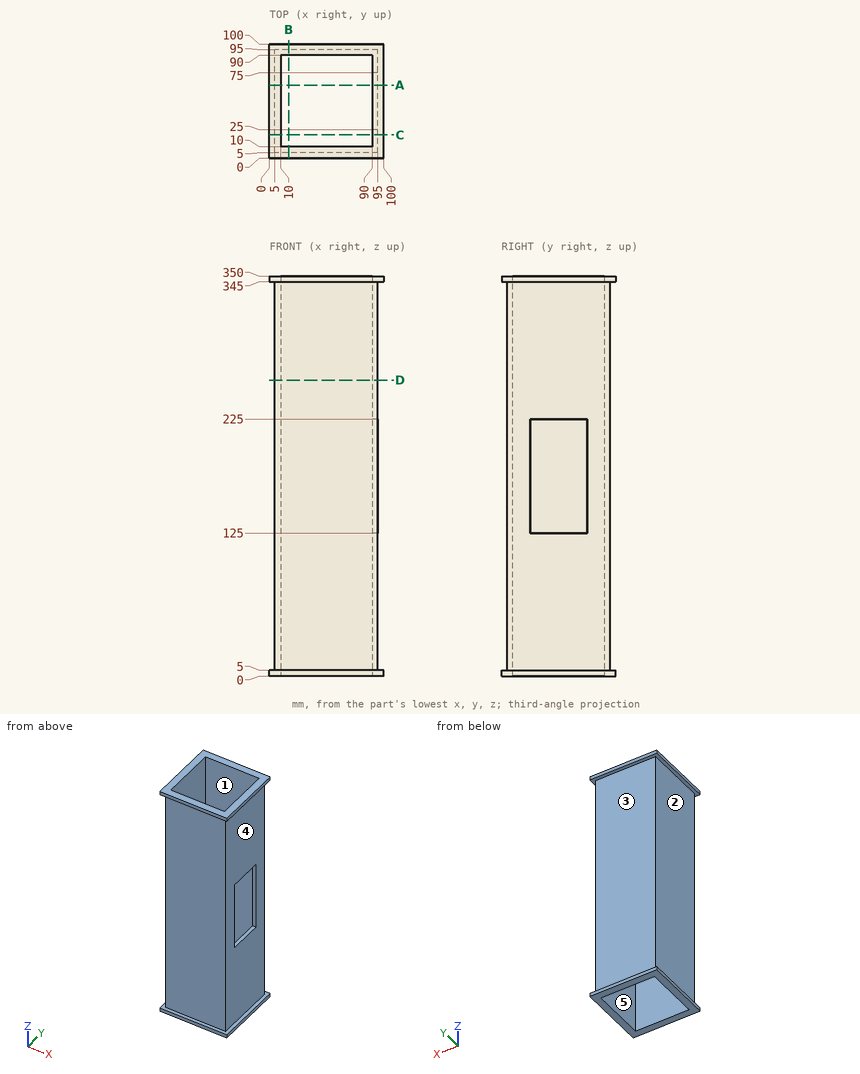
Job drawing, mm, ordinate dimensions from the low corner. One solid piece. A direction names the side the tool comes from. Give positions to 0.01 mm unless a question says otherwise; leave off trailing zeros. Loops run counter-clockwise (first coordinate to the right, second up) from the corner with the lowest first, then second, coordinate; pieces in that order, holes last. Notation, with made-up numbers: M 46,-31.75 L 69,-31.75 A13 ccw 69,-26.75 Z; hole C -5,67.25 d10. An arc over 180 degrees is marked long. Put each result on its own line as item: value. Start each with the question number.
1) Saw through at A-A (y = 64). List the corners of the cut face in (x, z), then the cut area to 3 significant figures.
2) Probe probe 1 along Z at (x, y) = (92, 42.5); probe 2 along Y at (x, z) = (37, 218.5). List the from-to ranges inside material, lowest first.
3) Pull direction Z, two halves, no side cores. Call the marked faces 4 and 5: +Z half, -Z half, draft (parallel to the pull), parting line (faces both ways), or undercut.
4) Saw through at B-B (x = 17). List the corners of the cut face in (y, z).
5) 3-axis set-ups, long thin cutter, end or side, ignore diameter. For the marked faces 1, 2 and 3: which of +Z, -Z, +X, -X, +Y, -Y reach the whole face in a straight line?
6) Flat gauge pins, fed straight in: pin 1 (2 mm diameter, centred on x = 35, z = 114, fed in from +Y); pin 2 (10 mm diameter, centred on y = 51.5, z = 245.5, fed in from -X); pin 3 (1.5 mm diameter, centred on y = 44, z = 314, fed in from +X). Where does each tip first touch, or does it go through?
7) Saw through at D-D (z = 259). List the corners of the cut face in (x, y).
Numbers:
1. outline: M 0,0 L 10,0 L 10,350 L 0,350 L 0,345 L 5,345 L 5,5 L 0,5 Z; M 90,0 L 100,0 L 100,5 L 95,5 L 95,125 L 90,125 Z; M 90,225 L 95,225 L 95,345 L 100,345 L 100,350 L 90,350 Z
1. area: 3,100 mm^2
2. probe 1: 0 to 125, 225 to 350
2. probe 2: 5 to 10, 90 to 95
3. face 4: undercut
3. face 5: draft
4. outline: M 0,0 L 10,0 L 10,350 L 0,350 L 0,345 L 5,345 L 5,5 L 0,5 Z; M 90,0 L 100,0 L 100,5 L 95,5 L 95,345 L 100,345 L 100,350 L 90,350 Z
5. face 1: +Z, -Z
5. face 2: -X, +Y, -Y
5. face 3: +X, -X, +Y
6. pin 1: y = 95
6. pin 2: x = 5
6. pin 3: x = 95
7. outline: M 5,5 L 95,5 L 95,95 L 5,95 Z; hole M 10,10 L 90,10 L 90,90 L 10,90 Z
